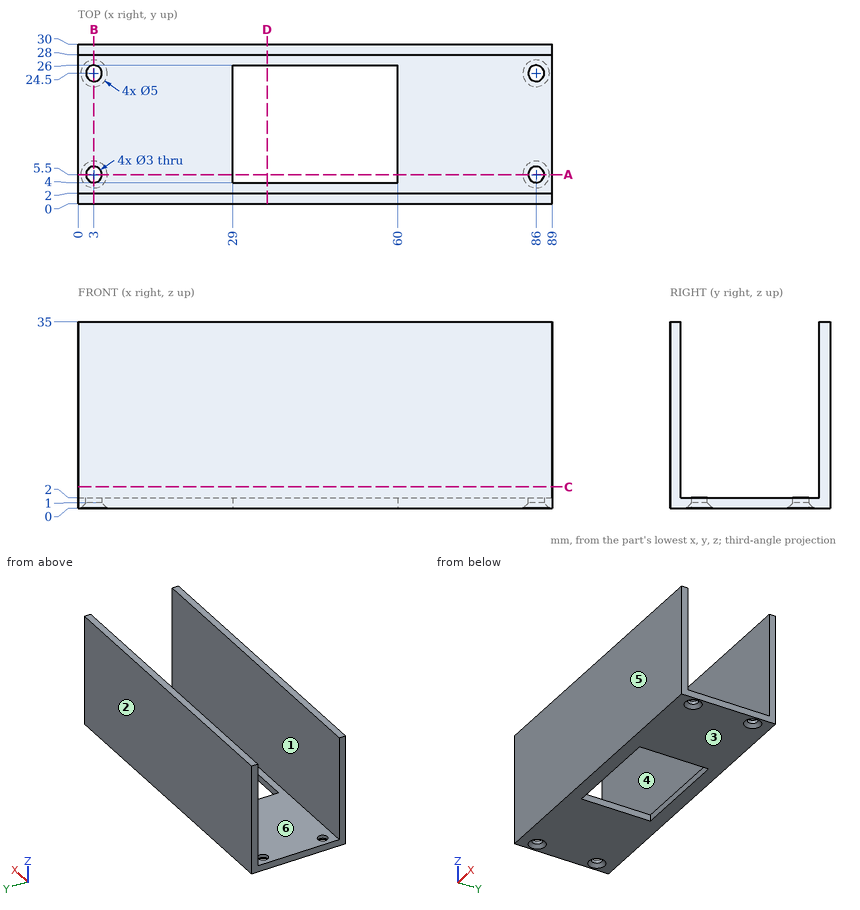
Can you work these out from the drawing? Everything is in mm from the part's minimum corner. A direction names the side the tool comes from. Coordinates: 2 decimals unless noted, no trailing zeros. Write each loop counter-clockwise with the first axis right and the second up, starting at its lowest first coordinate (ties: lowest second). Pieces come first, ordered by that corner, then holes. Notation, with made-up numbers: (-39.5, 68.25) -> (11.5, 68.25) arc R20 cw to (11.5, 97.25) -> close; hole circle Ø9 at (-3, 23.5). An arc over 180 degrees is marked (long way). Write item = value, one per line.
(1) Imagine slicing it at B-B (x = 3). Please give me the cut outline in (y, z).
Verdict:
outline = (0, 0) -> (3, 0) -> (4, 1) -> (4, 2) -> (2, 2) -> (2, 35) -> (0, 35) -> close; (7, 1) -> (8, 0) -> (22, 0) -> (23, 1) -> (23, 2) -> (7, 2) -> close; (26, 1) -> (27, 0) -> (30, 0) -> (30, 35) -> (28, 35) -> (28, 2) -> (26, 2) -> close
(2) If I drill on probe 1 along Y at (x, z) = (86, 1.6); probe 2 along Y at (x, z) = (74, 10.5); probe 3 along Z at (x, y) = (9, 23), over which ranges is the centre line in solid material (lowest first)?
Verdict:
probe_1 = 0 to 4, 7 to 23, 26 to 30
probe_2 = 0 to 2, 28 to 30
probe_3 = 0 to 2
(3) On a 3-axis mill with a long thin cutter (end or side, diameter ignored), from which of +Z, -Z, +X, -X, +Y, -Y can I reach the whole of each face in a straight line? I mean the marked faces 1 and 2. Say none if no direction works.
Verdict:
face_1 = +Z, +X, -X
face_2 = +Z, -Z, +X, -X, +Y
(4) Imagine slicing it at C-C (z = 4). Please give me the cut outline in (x, y), and give its area (3 significant figures).
Verdict:
outline = (0, 0) -> (89, 0) -> (89, 2) -> (0, 2) -> close; (0, 28) -> (89, 28) -> (89, 30) -> (0, 30) -> close
area = 356 mm^2
(5) Imagine slicing it at A-A (y = 5.5). Please give me the cut outline in (x, z), and give its area (3 significant figures).
Verdict:
outline = (0, 0) -> (0.5, 0) -> (1.5, 1) -> (1.5, 2) -> (0, 2) -> close; (4.5, 1) -> (5.5, 0) -> (29, 0) -> (29, 2) -> (4.5, 2) -> close; (60, 0) -> (83.5, 0) -> (84.5, 1) -> (84.5, 2) -> (60, 2) -> close; (87.5, 1) -> (88.5, 0) -> (89, 0) -> (89, 2) -> (87.5, 2) -> close
area = 102 mm^2
(6) For pin 1 (2.5 mm diameter, centred on x = 86, y = 24.5, fed in from -Z); pin 2 (3.5 mm diameter, centred on x = 3, y = 24.5, fed in from +Z), each with a flat end and sliding along its axis, tell me the tip position at first contact or that it passes through.
Verdict:
pin_1 = through
pin_2 = 2
(7) Thinking about a two-plate mould opening in Y: for the marked faces 3, 4, 5 and 6, which applies, +Y half, -Y half, draft (parallel to the pull), parting line (faces both ways), or undercut?
Verdict:
face_3 = draft
face_4 = undercut
face_5 = -Y half
face_6 = undercut
(8) Imagine slicing it at D-D (x = 35.5). Please give me the cut outline in (y, z), and give its area (3 significant figures).
Verdict:
outline = (0, 0) -> (4, 0) -> (4, 2) -> (2, 2) -> (2, 35) -> (0, 35) -> close; (26, 0) -> (30, 0) -> (30, 35) -> (28, 35) -> (28, 2) -> (26, 2) -> close
area = 148 mm^2
